```python
from build123d import *

# Parameters (mm, degrees)
SKETCH1_R           = 15
BOSS_EXTRUDE3_DEPTH = 2
SKETCH2_R           = 14.25
SKETCH2_R_2         = 13.5
BOSS_EXTRUDE4_DEPTH = 3
SKETCH6_R           = 0.5


with BuildPart() as part:
    # Sketch1 → Boss-Extrude3 (new body)
    with BuildSketch(Plane(origin=(0, 0, 0), x_dir=(1, 0, 0), z_dir=(0, 1, 0))):
        with Locations(Location((0, 0, 0), (0, 0, 270))):
            Circle(SKETCH1_R)
    extrude(amount=BOSS_EXTRUDE3_DEPTH)

    # Sketch2 → Boss-Extrude4 (add)
    with BuildSketch(Plane(origin=(0, 2, 0), x_dir=(1, 0, 0), z_dir=(0, 1, 0))):
        with Locations(Location((0, 0, 0), (0, 0, 270))):
            Circle(SKETCH2_R)
        with Locations(Location((0, 0, 0), (0, 0, 270))):
            Circle(SKETCH2_R_2, mode=Mode.SUBTRACT)
    extrude(amount=BOSS_EXTRUDE4_DEPTH)

    # Sweep1: sweep along a path in Sketch7
    with BuildLine(Plane(origin=(0, 0, 0), x_dir=(0, 0, -1), z_dir=(1, 0, 0))) as sweep1_path:
        Line((-3.5, 0), (-3.5, -1))
        ThreePointArc((-3.5, -1), (-3.207106781, -1.707106781), (-2.5, -2))
        Line((-2.5, -2), (2.5, -2))
        ThreePointArc((2.5, -2), (3.207106781, -1.707106781), (3.5, -1))
        Line((3.5, -1), (3.5, 0))
    # Sketch6 → Sweep1 (sweep)
    with BuildSketch(Plane.XZ):
        with Locations((0, 3.5)):
            Circle(SKETCH6_R)
    sweep(path=sweep1_path.line)


solid = part.part
```
The listing builds one solid part. Answer for the finished solid, in the listing's coordinates (mm). A direction names the side the tool comes from. Give positions to 0.01 mm unless a question says otherwise; leave off trailing zeros. Order: outer loops, then holes, each group sorted by start corner. A loop starts at its lowest first (then second) coordinate and runs counter-clockwise, first axis right, second up.
1) Find section D-D on z = -10.75. Write down the section's boundary in (x, y), then the cut area to 3 significant figures.
Reported:
outline: (-10.46, 0) - (10.46, 0) - (10.46, 2) - (9.35, 2) - (9.35, 5) - (8.17, 5) - (8.17, 2) - (-8.17, 2) - (-8.17, 5) - (-9.35, 5) - (-9.35, 2) - (-10.46, 2) - close
area: 49.0 mm2
2) For faces 1 (the face through (-0.065, -0.507, 3.996)), 2 (the face through (-12, 2, 8)), determine the directions among +Z, -Z, +X, -X, +Y, -Y from which every point of the face is accessible in a straight line to the end or side of a thin tool.
Reported:
face 1: none
face 2: +Y
3) Given P1, Ø1.5, axis at y = 0.5, z = 10, coming from the -X side; P2, Ø2, axis at x = -11, y = 1, coming from the +Z side; P3, Ø2, axis at x = 8.5, y = -0.5, coming from the -Z side, each flat-ended and moving along its own axis, determine where each tip first touches the part or whether it passes through.
Reported:
P1: stops at x = -11.81
P2: stops at z = 11.18
P3: stops at z = -12.91
4) Find section B-B on x = 0. Write down the section's boundary in (y, z), then the cut area to 3 significant figures.
Reported:
outline: (-2.5, -2.5) arc R1.5 ccw to (-1, -4) - (0, -4) - (0, -15) - (2, -15) - (2, -14.25) - (5, -14.25) - (5, -13.5) - (2, -13.5) - (2, 13.5) - (5, 13.5) - (5, 14.25) - (2, 14.25) - (2, 15) - (0, 15) - (0, 4) - (-1, 4) arc R1.5 ccw to (-2.5, 2.5) - close; hole (-1.5, -2.5) arc R0.5 ccw to (-1, -3) - (0, -3) - (0, 3) - (-1, 3) arc R0.5 ccw to (-1.5, 2.5) - close
area: 74.6 mm2
5) Find section A-A on z = 0. Write down the section's boundary in (x, y).
Reported:
outline: (-15, 0) - (15, 0) - (15, 2) - (14.25, 2) - (14.25, 5) - (13.5, 5) - (13.5, 2) - (-13.5, 2) - (-13.5, 5) - (-14.25, 5) - (-14.25, 2) - (-15, 2) - close; circle Ø1 at (0, -2)
6) Find section C-C on y = 3.5. Write down the section's boundary in (x, z), then the cut area to 3 significant figures.
Reported:
outline: circle Ø28.5 at (0, 0); hole circle Ø27 at (0, 0)
area: 65.4 mm2
7) Determine the mould class of faces 3 (the face through (0.66, 0.986, -14.985)), 4 (the face through (-0.065, -0.493, -3.996)), 5 (the face through (-5, 5, 13)), 6 (the face through (-0.065, -2.496, -0.035)) for opening direction Z: pulls with the +Z half, pulls with the -Z half, needs draft (parallel to the pull), parting line crosses it, or undercut.
Reported:
face 3: parting line crosses it
face 4: undercut
face 5: needs draft
face 6: undercut
8) Consider line 1 along Y through (x, z) = (0, -1.5); line 2 along X through (y, z) = (4, 0); line 3 along Y through (x, z) = (3.25, 5.75). Determine where each line is inside the solid, lowest interval first.
Reported:
line 1: y = -2.5 to -1.5, 0 to 2
line 2: x = -14.25 to -13.5, 13.5 to 14.25
line 3: y = 0 to 2
